```python
from build123d import *

# Parameters (mm, degrees)
SALIENTE_EXTRUIR1_DEPTH = 0.5
SALIENTE_EXTRUIR2_DEPTH = 3


with BuildPart() as part:
    # Croquis1 → Saliente-Extruir1 (new body)
    with BuildSketch(Plane(origin=(0, 0, 0), x_dir=(1, 0, 0), z_dir=(0, 1, 0))):
        Polygon((0, 0), (0, 2.5), (4.5, 2.5), (4.5, 7), (7, 7), (7, 0), align=None)
    extrude(amount=SALIENTE_EXTRUIR1_DEPTH)

    # Croquis2 → Saliente-Extruir2 (add)
    with BuildSketch(Plane(origin=(0, 0.5, 0), x_dir=(1, 0, 0), z_dir=(0, 1, 0))):
        Polygon((0, 2.5), (0, 0), (0, -2), (9, -2), (9, 7), (7, 7), (4.5, 7), (4.5, 2.5), align=None)
    extrude(amount=SALIENTE_EXTRUIR2_DEPTH)


solid = part.part
```
CAD build for the part. Positions are in the model's coordinates, mm. A direction names the side the tool comes from. Round coordinates to 2 decimals unless told otherwise and drop trailing zeros. Write each loop counter-clockwise with the first axis right and the second up, starting at its lowest first coordinate (ties: lowest second). Pieces come first, ordered by that corner, then holes. Notation, with made-up numbers: (57, 58.5) - (114, 58.5) arc R23 cw to (114, 71.5) - close; hole circle Ø9 at (46, 53.25). An arc over 180 degrees is marked (long way). Return JSON: item names as keys, results as strings. Group by question number.
Item 1: Band-saw the part on A-A on y = 2.95. List the corners of the cut face in (x, z).
Item 2: Band-saw the part on B-B on x = 5.5. List the corners of the cut face in (y, z), plus the area to 3 significant figures.
Item 3: Flat gauge pins, fed straight in: pin 1 Ø2.5 at (x, z) = (4.5, -0.5) entering from -Y; pin 2 Ø1.8 at (y, z) = (1.5, -4) entering from -X; pin 3 Ø1.8 at (x, y) = (3, 2.5) entering from -Z. Where does each tip first touch, or does it go through?
Item 4: Band-saw the part on D-D on x = 8. List the corners of the cut face in (y, z).
Item 5: 3-axis set-ups, long thin cutter, end or side, ignore diameter. For faces 1 (the face through (0, 2, 0)), 2 (the face through (4.5, 2, -5)): which of +Z, -Z, +X, -X, +Y, -Y reach the whole face in a straight line?
Item 6: Probe probe 1 along X at (y, z) = (2.2, -6.25); probe 2 along Z at (x, y) = (4, 1.3); probe 3 along Y at (x, z) = (7.25, 0.75). List the from-to ranges inside material, lowest first.
Item 7: Band-saw the part on C-C on z = 1.25. List the corners of the cut face in (x, y).
Resolved:
{
 "1": {"outline": "(0, -2.5) - (4.5, -2.5) - (4.5, -7) - (9, -7) - (9, 2) - (0, 2) - close"},
 "2": {"outline": "(0, -7) - (3.5, -7) - (3.5, 2) - (0.5, 2) - (0.5, 0) - (0, 0) - close", "area": "30.5 mm²"},
 "3": {"pin 1": "stops at y = 0", "pin 2": "stops at x = 4.5", "pin 3": "stops at z = -2.5"},
 "4": {"outline": "(0.5, -7) - (3.5, -7) - (3.5, 2) - (0.5, 2) - close"},
 "5": {"face 1": "+Z, -Z, -X, +Y, -Y", "face 2": "-Z, -X, +Y, -Y"},
 "6": {"probe 1": "x = 4.5 to 9", "probe 2": "z = -2.5 to 2", "probe 3": "y = 0.5 to 3.5"},
 "7": {"outline": "(0, 0.5) - (9, 0.5) - (9, 3.5) - (0, 3.5) - close"}
}
